Work out the finished part from the listing and answer in its coordinate system (mm). A direction names the side the tool comes from. Give positions to 0.01 mm unless a question says otherwise; leave off trailing zeros.
Autodesk Inventor part; units mm, degrees
ref_plane "YZ Plane" through (0, 0, 0) normal (1, 0, 0) x (0, 1, 0)
ref_plane "XZ Plane" through (0, 0, 0) normal (0, 1, 0) x (-1, 0, 0)
ref_plane "XY Plane" through (0, 0, 0) normal (0, 0, 1) x (1, 0, 0)
sketch "Sketch1" plane through (0, 0, 0) normal (0, 0, 1) x (1, 0, 0)
  line L0 (0, 0) -> (114.3, 0)
  line L1 (114.3, 0) -> (114.3, 38.1)
  line L2 (114.3, 38.1) -> (-38.1, 38.1)
  line L3 (-38.1, 38.1) -> (-38.1, -88.9)
  line L4 (-38.1, -88.9) -> (0, -88.9)
  line L5 (0, -88.9) -> (0, 0)
  dimension "d0" = 152.4
  dimension "d1" = 127
  dimension "d2" = 38.1
  dimension "d3" = 38.1
extrude "Extrusion1" add sketch "Sketch1" along normal mid plane 50.8
fillet "Fillet1" radius 38.1 3 edges at (0, -88.9, 0) (114.3, 0, 0) (0, 0, 0)
fillet "Fillet2" radius 25.4 8 edges at (0, -44.45, 25.4) (-11.1591, -77.7409, 25.4) (57.15, 0, 25.4) (103.1409, 11.1591, 25.4) (57.15, 0, -25.4) (103.1409, 11.1591, -25.4) (-11.1591, -77.7409, -25.4) (0, -44.45, -25.4)
properties part number "shelfBracket"
Item 1: Flat-ended cylindrical pins translate along their axes: pin 1 Ø12 at (x, y) = (35, 5) entering from +Z; pin 2 Ø5 at (y, z) = (-18.5, 5) entering from +X; pin 3 Ø12 at (y, z) = (-25, 8) entering from +X. Find the tip coordinate at first contact, or state that the pin passes through.
Item 2: Consider line 1 (X direction, y = -13.5, z = 22.5); line 2 (Y direction, x = 73, z = 23); line 3 (Y direction, x = 58, z = -10). Determine where each line is inside the solid, lowest interval first.
Item 3: For faces 1 (the face through (39, 38.1, 0)), 2 (the face through (57.42, 7.24, -17.76)), 3 (the face through (-7.64, -44.36, 18.16)), determine the directions among +Z, -Z, +X, -X, +Y, -Y from which every point of the face is accessible in a straight line to the end or side of a thin tool.
Ans:
1. pin 1: stops at z = 21
1. pin 2: stops at x = 6.55
1. pin 3: stops at x = 4.13
2. line 1: x = -38.1 to -7.39
2. line 2: y = 14.62 to 38.1
2. line 3: y = 2.05 to 38.1
3. face 1: +Z, -Z, +X, -X, +Y
3. face 2: -Z, +X, -Y
3. face 3: +Z, +X, -Y
